Model file for the job. Use its own axes, mm. Face numbers are marked on the shaded views. A direction names the side the tool comes from. Coordinates: 2 decimals unless noted, no trailing zeros. Order: outer loops, then holes, each group sorted by start corner. A loop starts at its lowest first (then second) coordinate and runs counter-clockwise, first axis right, second up.
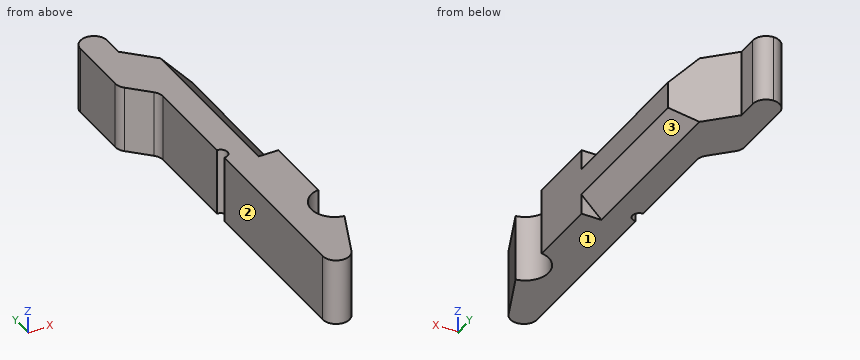
Autodesk Fusion 360 part; units mm, degrees
sketch "Sketch1" plane through (0, 0, 0) normal (0, 0, 1) x (1, 0, 0)
  circle A0 centre (0, 0) radius 3.5
  line L0 (-11.5, 49) -> (-11.5, 37)
  line L1 (-0.5, -3.4641) -> (-0.5, 37)
  line L2 (-0.5, -3.4641) -> (-7.5, -20)
  circle A1 centre (-7.5, 16.9115) radius 1
  line L3 (-11.5, 49) -> (-7.5, 49)
  line L4 (-11.5, 37) -> (-7.5, 33)
  line L5 (-7.5, 44) -> (-0.5, 37)
  line L6 (-7.5, -20) -> (-7.5, 33)
  line L7 (-7.5, 44) -> (-7.5, 49)
  point P0 (-7.5, 16.9115)
  dimension "d1" = 7
  dimension "d2" = 4
  dimension "d6" = 0.5
  dimension "d7" = 20
  dimension "d8" = 7
  dimension "d9" = 18.5
  dimension "d10" = 2
  dimension "d11" = 69
  dimension "d12" = 12
  dimension "d14" = 5
  dimension "d26" = 45
extrude "Extrude1" add sketch "Sketch1" along normal blind 10 contours A0 L0 L1 L2 A1 L3 L4 L5 L6 L7
sketch "Sketch2" plane through (0, 49, 0) normal (0, 1, 0) x (-1, 0, 0)
  line L0 (7.5, 0) -> (11.5, 0)
  line L1 (11.5, 0) -> (11.5, 10)
  line L2 (11.5, 10) -> (7.5, 10)
  line L3 (7.5, 10) -> (7.5, 0)
  line L4 (3.5, 0) -> (-1.5, 5)
  line L5 (-1.5, 5) -> (3.5, 10)
  line L6 (7.5, 0) -> (0.5, 0)
  line L7 (3.5, 10) -> (-2, 10)
  line L8 (-2, 10) -> (-2, 0)
  line L9 (-2, 0) -> (3.5, 0)
  line L10 (0.5, 10) -> (7.5, 10)
  point P0 (0.5, 0)
  point P1 (0.5, 10)
  dimension "d17" = 3
  dimension "d18" = 3
  dimension "d19" = 45
extrude "Extrude2" cut sketch "Sketch2" against normal blind 35 contours L4 L5 L6 L7 L8 L9 L10
fillet "Fillet1" radius 2 2 edges at (-11.5, 49, 5) (-7.5, 49, 5)
fillet "Fillet2" radius 2 3 edges at (-7.5, 33, 5) (-11.5, 37, 5) (-7.5, -20, 5)
Q1. Drop flat-ended pins along their axis: P1, Ø4, axis at x = -2.5, z = 1.5, coming from the -Y side; P2, Ø1, axis at y = 23.5, z = 2.5, coming from the -X side; P3, Ø1.5, axis at x = -1.5, z = 2, coming from the +Y side. Give the stop position or say it passes through.
Established:
P1: stops at y = -11.88
P2: stops at x = -7.5
P3: stops at y = 38.75
Q2. Probe line 1 (Y direction, x = -0.75, z = 3); line 2 (X direction, y = 19, z = 4.75); line 3 (Y direction, x = -1.75, z = 1.5). List the from-to ranges inside material, lowest first.
Established:
line 1: y = -4.05 to -3.42, 3.42 to 37.25
line 2: x = -7.5 to -0.5
line 3: y = -6.42 to -3.03, 3.03 to 14
Q3. Cut at B-B, the plane y = 27. List the corners of the cut face in (x, z).
Established:
outline: (-7.5, 0) - (-3.5, 0) - (-0.5, 3) - (-0.5, 7) - (-3.5, 10) - (-7.5, 10) - close
Q4. Which spindle directions (+Z, -Z, +X, -X, +Y, -Y) get a long thin tool onto all of the face, cutting with end or side? Do the marked faces 1, 2 and 3. Say none if no direction does.
Established:
face 1: -Z, +X, -X, +Y, -Y
face 2: +Z, -Z, -X, -Y
face 3: -Z, +X, +Y
Q5. Cut at D-D, the plane x = -5.25. List the corners of the cut face in (y, z), plus the area to 3 significant figures.
Established:
outline: (-12.13, 0) - (41.75, 0) - (41.75, 10) - (-12.13, 10) - close
area: 539 mm2
